The listing builds one solid part. Answer for the finished solid, in the listing's coordinates (mm). Face numbers are marked on the shaded views. A direction names the side the tool comes from. Coordinates: 2 decimals unless noted, no trailing zeros. Loops run counter-clockwise (first coordinate to the right, second up) from the corner with the lowest first, then second, coordinate; pieces in that order, holes last. Notation, with made-up numbers: M -29,49.5 L 17,49.5 A30 cw 17,84.5 Z; hole C 37.5,-30.5 d3. An arc over 180 degrees is marked long. Return JSON: item names as keys, results as strings. Group by question number.
1. Section C-C (x = -4.75) is taken. Write down the section's boundary in (y, z).
2. Straight lines are drawn through the part: L1, parallel to X at y = 0, z = 0; L2, parallel to Y at x = 1.75, z = -7.5. For each, find the intervals that lie inside material, in ascending order. Write a range as from..to.
3. Section A-A (z = 0) is taken. Write down the section's boundary in (x, y), then the cut area to 3 significant figures.
4. Given P1, Ø8, axis at x = 5.5, z = -6.5, coming from the -Y side, flat-ended and moving along its own axis, determine where the tip first touches the part or whether it passes through.
5. Section B-B (x = 0) is taken. Write down the section's boundary in (y, z).
6. Which of the six approach directions +Z, -Z, +X, -X, +Y, -Y give full straight-line access (tool end or side, diameter ignored) to the marked faces 1 and 2?
7. The mould has two halves that part along Z. Classify the marked faces 3, 4 and 5: pulls with the +Z half, pulls with the -Z half, needs draft (parallel to the pull), parting line crosses it, or undercut.
8. Section D-D (z = 5.5) is taken. Write down the section's boundary in (x, y).
```python
from build123d import *

# Parameters (mm, degrees)
SKETCH1_R           = 11
SKETCH1_R_2         = 4
BOSS_EXTRUDE1_DEPTH = 3.5
SKETCH2_R           = 10
SKETCH2_R_2         = 6
CUT_EXTRUDE1_DEPTH  = 0.1


with BuildPart() as part:
    # Sketch1 → Boss-Extrude1 (new body, symmetric)
    with BuildSketch(Plane(origin=(0, 0, 0), x_dir=(1, 0, 0), z_dir=(0, 1, 0))):
        Circle(SKETCH1_R)
        Circle(SKETCH1_R_2, mode=Mode.SUBTRACT)
    extrude(amount=BOSS_EXTRUDE1_DEPTH, both=True)

    # Sketch2 → Cut-Extrude1 (cut)
    with BuildSketch(Plane(origin=(0, 3.5, 0), x_dir=(1, 0, 0), z_dir=(0, 1, 0))):
        Circle(SKETCH2_R)
        Circle(SKETCH2_R_2, mode=Mode.SUBTRACT)
    cut_extrude1 = extrude(amount=-CUT_EXTRUDE1_DEPTH, mode=Mode.SUBTRACT)

    # Mirror1: Cut-Extrude1 across plane
    add(cut_extrude1.mirror(Plane.ZX), mode=Mode.SUBTRACT)


solid = part.part
```
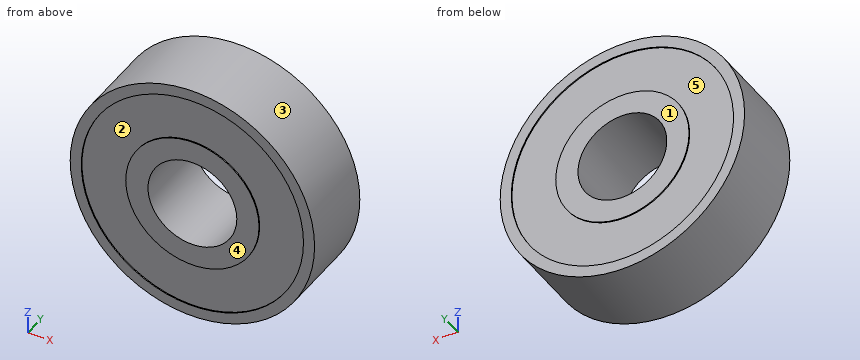
Worked out:
{
 "1": {"outline": "M -3.5,-9.92 L 3.5,-9.92 L 3.5,-8.8 L 3.4,-8.8 L 3.4,-3.67 L 3.5,-3.67 L 3.5,3.67 L 3.4,3.67 L 3.4,8.8 L 3.5,8.8 L 3.5,9.92 L -3.5,9.92 L -3.5,8.8 L -3.4,8.8 L -3.4,3.67 L -3.5,3.67 L -3.5,-3.67 L -3.4,-3.67 L -3.4,-8.8 L -3.5,-8.8 Z"},
 "2": {"L1": "-11..-4, 4..11", "L2": "-3.4..3.4"},
 "3": {"outline": "M -11,-3.5 L -10,-3.5 L -10,-3.4 L -6,-3.4 L -6,-3.5 L -4,-3.5 L -4,3.5 L -6,3.5 L -6,3.4 L -10,3.4 L -10,3.5 L -11,3.5 Z; M 4,-3.5 L 6,-3.5 L 6,-3.4 L 10,-3.4 L 10,-3.5 L 11,-3.5 L 11,3.5 L 10,3.5 L 10,3.4 L 6,3.4 L 6,3.5 L 4,3.5 Z", "area": "96.4 mm^2"},
 "4": {"P1": "y = -3.5"},
 "5": {"outline": "M -3.5,-11 L 3.5,-11 L 3.5,-10 L 3.4,-10 L 3.4,-6 L 3.5,-6 L 3.5,-4 L -3.5,-4 L -3.5,-6 L -3.4,-6 L -3.4,-10 L -3.5,-10 Z; M -3.5,4 L 3.5,4 L 3.5,6 L 3.4,6 L 3.4,10 L 3.5,10 L 3.5,11 L -3.5,11 L -3.5,10 L -3.4,10 L -3.4,6 L -3.5,6 Z"},
 "6": {"face 1": "+Z, -Z, +X, -X, +Y", "face 2": "-Y"},
 "7": {"face 3": "parting line crosses it", "face 4": "needs draft", "face 5": "undercut"},
 "8": {"outline": "M -9.53,-3.5 L -8.35,-3.5 L -8.35,-3.4 L -2.4,-3.4 L -2.4,-3.5 L 2.4,-3.5 L 2.4,-3.4 L 8.35,-3.4 L 8.35,-3.5 L 9.53,-3.5 L 9.53,3.5 L 8.35,3.5 L 8.35,3.4 L 2.4,3.4 L 2.4,3.5 L -2.4,3.5 L -2.4,3.4 L -8.35,3.4 L -8.35,3.5 L -9.53,3.5 Z"}
}
